from build123d import *

# Parameters (mm, degrees)
SKETCH1_R           = 2.25
BOSS_EXTRUDE1_DEPTH = 15
SKETCH2_R           = 0.25
SKETCH4_R           = 0.1
FILLET1_R           = 0.2


with BuildPart() as part:
    # Sketch1 → Boss-Extrude1 (new body)
    with BuildSketch(Plane(origin=(0, 0, 0), x_dir=(1, 0, 0), z_dir=(0, 1, 0))):
        with Locations(Location((0, 0, 0), (0, 0, 270))):
            Circle(SKETCH1_R)
    extrude(amount=BOSS_EXTRUDE1_DEPTH)

    # Sweep1: sweep along a path in Sketch3
    with BuildLine(Plane(origin=(0, 0, 0), x_dir=(0, 0, -1), z_dir=(1, 0, 0))) as sweep1_path:
        Line((0, 0), (0, -1.1))
        ThreePointArc((0, -1.1), (0.175735931, -1.524264069), (0.6, -1.7))
        Line((0.6, -1.7), (3.35, -1.7))
    # Sketch2 → Sweep1 (sweep)
    with BuildSketch(Plane.XZ):
        Circle(SKETCH2_R)
    sweep(path=sweep1_path.line)

    # Sweep2: sweep along a path in Sketch5
    with BuildLine(Plane(origin=(0, 0, 0), x_dir=(0, 0, -1), z_dir=(1, 0, 0))) as sweep2_path:
        Line((0, 0), (0, -1.1))
        ThreePointArc((0, -1.1), (0.175735931, -1.524264069), (0.6, -1.7))
        Line((0.6, -1.7), (1.1, -1.7))
    # Sketch4 → Sweep2 (sweep)
    with BuildSketch(Plane.XZ):
        with Locations((-1.125, 0)):
            Circle(SKETCH4_R)
    sweep(path=sweep2_path.line)

    # Fillet1
    fillet1_edges = [part.edges().sort_by_distance(p)[0] for p in [
        (0, 15, -2.25),
    ]]
    fillet(fillet1_edges, radius=FILLET1_R)


solid = part.part
Geometry check sheet. Reference: the model listing, model coordinates, mm. Round coordinates to 2 decimals unless told otherwise and drop trailing zeros. Order: outer loops, then holes, each group sorted by start corner. A loop starts at its lowest first (then second) coordinate and runs counter-clockwise, first axis right, second up. Notation, with made-up numbers: (21, 89) - (68, 89) arc R31 ccw to (68, 125) - close; hole circle Ø4 at (-22.5, -8.75). An arc over 180 degrees is marked (long way). One line per question, with ' | ' between items. Start each with the question number.
(1) Thickness scan on L1, parallel to Y at x = 0.4, z = -0.6; L2, parallel to Z at x = 0.05, y = 2; L3, parallel to X at y = 1.5, z = -0.55. Record the ranges inside material, lowest first. Write a range as [from, to].
(2) Sectioned sample at B-B on y = 10.5. Record the cut outline in (x, z), and give its area (3 significant figures).
(3) Sectioned sample at A-A on x = 0. Record the cut outline in (y, z), and give its area (3 significant figures).
(4) Depth check by flat-ended pin: pin 1 Ø3 at (y, z) = (6.5, 1.5) entering from -X. Enter the tip coordinate at first touch or a pass-through.
Conclusion:
1) L1: y = [0, 15] | L2: z = [-2.25, 2.25] | L3: x = [-2.18, 2.18]
2) outline: circle Ø4.5 at (0, 0) | area: 15.9 mm2
3) outline: (-1.95, -3.35) - (-1.45, -3.35) - (-1.45, -0.6) arc R0.35 cw to (-1.1, -0.25) - (0, -0.25) - (0, -2.25) - (14.8, -2.25) arc R0.2 ccw to (15, -2.05) - (15, 2.05) arc R0.2 ccw to (14.8, 2.25) - (0, 2.25) - (0, 0.25) - (-1.1, 0.25) arc R0.85 ccw to (-1.95, -0.6) - close | area: 69.9 mm2
4) pin 1: stops at x = -2.25
